Can you work these out from the model? Positions are in its coordinate system, mm. Coordinates: 2 decimals unless noted, no trailing zeros. Order: outer loops, then holes, each group sorted by start corner. A loop starts at its lowest first (then second) coordinate and runs counter-clockwise, first axis right, second up. Notation, with made-up numbers: M 19.25,-22.75 L 69.25,-22.75 A17 cw 69.25,-4.75 Z; hole C 12,67.5 d7. An arc over 180 degrees is marked long. Answer as CSV lines item,"result". Start each with the question number.
1. If we section it at A-A (x = -6): List the corners of the cut face in (y, z) for me.
2. If we section it at D-D (z = 0): List the corners of the cut face in (x, y) for me, plus the area to 3 significant figures.
3. If we section it at B-B (y = 3.5): Give the number of separate pieces and of enclosed holes in the cut face, plus the area to 3 significant figures.
4. If we section it at C-C (z = 28.5): List the corners of the cut face in (x, y) for me, plus the area to 3 significant figures.
5. Will this pin go through, and if not, where does the flat tip stop? pin 1 (8 mm diameter, centred on x = 3.5, z = 25.5, fed in from -Y).
6. I need wall thicknesses on line 1 along Z through (x, y) = (5, 3.7); line 2 along Z through (x, y) = (-0.75, 0.75); line 3 along Z through (x, y) = (-5.5, 1.9). Which ranges of each line are inside material? Lowest first, please. Write a range as from..to.
```python
from build123d import *

# Parameters (mm, degrees)
SKETCH1_W                  = 20
SKETCH1_H                  = 120
BOSS_EXTRUDE1_DEPTH        = 5
F_3_3_3_3_DIAMETER_HOLE1_D = 3.3
SKETCH5_W                  = 5.1
SKETCH5_H                  = 5
SKETCH5_W_2                = 5
SKETCH5_H_2                = 5.1
CUT_EXTRUDE1_DEPTH         = 6
F_4_5_4_5_DIAMETER_HOLE2_D = 4.5


with BuildPart() as part:
    # Sketch1 → Boss-Extrude1 (new body)
    with BuildSketch(Plane(origin=(0, 0, 0), x_dir=(1, 0, 0), z_dir=(0, 1, 0))):
        Rectangle(SKETCH1_W, SKETCH1_H)
    extrude(amount=BOSS_EXTRUDE1_DEPTH)

    # Ø3.3 (3.3) Diameter Hole1 (through all)
    with Locations(Plane(origin=(0, 5, 0), x_dir=(1, 0, 0), z_dir=(0, 1, 0))):
        with Locations((5, 45), (5, -45)):
            Hole(F_3_3_3_3_DIAMETER_HOLE1_D / 2)

    # Sketch5 → Cut-Extrude1 (cut, through all)
    with BuildSketch(Plane(origin=(0, 5, 0), x_dir=(1, 0, 0), z_dir=(0, 1, 0))):
        with Locations((-5.45, 50)):
            Rectangle(SKETCH5_W, SKETCH5_H)
        with Locations((-5.45, -50)):
            Rectangle(SKETCH5_W, SKETCH5_H)
        with Locations((0, -55.45)):
            Rectangle(SKETCH5_W_2, SKETCH5_H_2)
        with Locations((0, 55.45)):
            Rectangle(SKETCH5_W_2, SKETCH5_H_2)
        with Locations((-5.45, 0)):
            Rectangle(SKETCH5_W, SKETCH5_H)
    extrude(amount=-CUT_EXTRUDE1_DEPTH, mode=Mode.SUBTRACT)

    # Ø4.5 (4.5) Diameter Hole2 (through all)
    with Locations(Plane(origin=(0, 5, 0), x_dir=(1, 0, 0), z_dir=(0, 1, 0))):
        with Locations((5, 28.5), (2, 0), (5, -28.5)):
            Hole(F_4_5_4_5_DIAMETER_HOLE2_D / 2)


solid = part.part
```
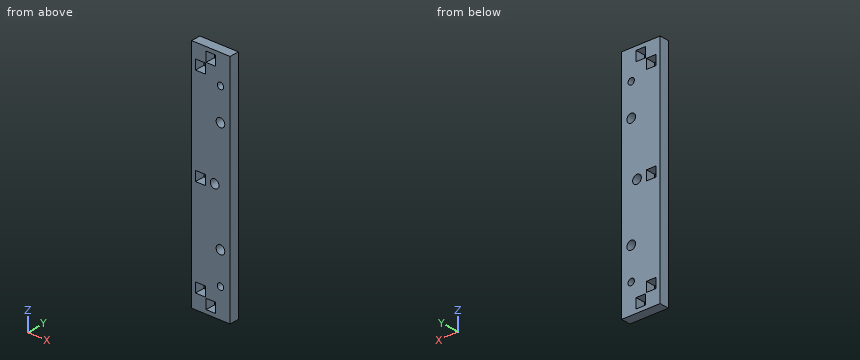
Solved:
1,outline,"M 0,-60 L 5,-60 L 5,-52.5 L 0,-52.5 Z; M 0,-47.5 L 5,-47.5 L 5,-2.5 L 0,-2.5 Z; M 0,2.5 L 5,2.5 L 5,47.5 L 0,47.5 Z; M 0,52.5 L 5,52.5 L 5,60 L 0,60 Z"
2,outline,"M -10,0 L -8,0 L -8,5 L -10,5 Z; M -2.9,0 L -0.25,0 L -0.25,5 L -2.9,5 Z; M 4.25,0 L 10,0 L 10,5 L 4.25,5 Z"
2,area,"52.0 mm²"
3,separate pieces,"1"
3,enclosed holes,"10"
3,area,"2,210 mm²"
4,outline,"M -10,0 L 2.75,0 L 2.75,5 L -10,5 Z; M 7.25,0 L 10,0 L 10,5 L 7.25,5 Z"
4,area,"77.5 mm²"
5,pin 1,"y = 0"
6,line 1,"-60..-46.65, -43.35..-30.75, -26.25..26.25, 30.75..43.35, 46.65..60"
6,line 2,"-60..-58, -52.9..52.9, 58..60"
6,line 3,"-60..-52.5, -47.5..-2.5, 2.5..47.5, 52.5..60"
